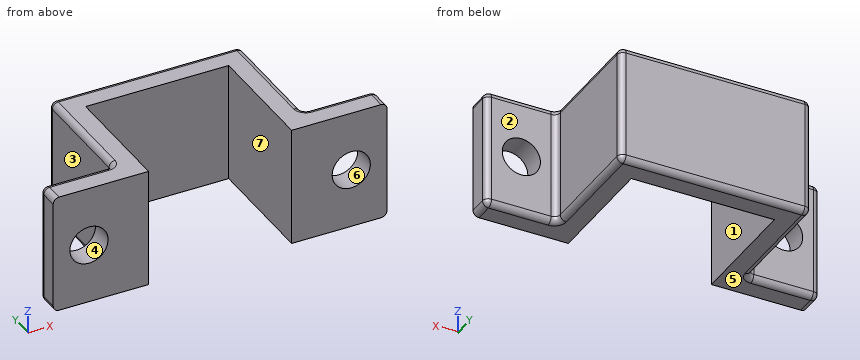
```python
from build123d import *

# Parameters (mm, degrees)
GRUNDK_RPER_DEPTH      = 10
SKIZZE2_W              = 12
SKIZZE2_H              = 10
AUSSCHNITT_MITTE_DEPTH = 21.976176963
SKIZZE3_R              = 1.6
BOHRUNGEN_DEPTH        = 20.899748742
VERRUNDUNG1_R          = 0.5


with BuildPart() as part:
    # Skizze1 → Grundkörper (new body)
    with BuildSketch(Plane.XY):
        Polygon((14, 0), (-14, 0), (-14, 2), (-8, 2), (-8, 12), (8, 12), (8, 2), (14, 2), align=None)
    extrude(amount=GRUNDK_RPER_DEPTH)

    # Skizze2 → Ausschnitt_Mitte (cut, through all)
    with BuildSketch(Plane.XY.offset(10)):
        with Locations((0, 5)):
            Rectangle(SKIZZE2_W, SKIZZE2_H)
    extrude(amount=-AUSSCHNITT_MITTE_DEPTH, mode=Mode.SUBTRACT)

    # Skizze3 → Bohrungen (cut, through all)
    with BuildSketch(Plane(origin=(0, 2, 0), x_dir=(1, 0, 0), z_dir=(0, 1, 0))):
        with Locations(Location((-11, -5, 0), (0, 0, 270))):
            Circle(SKIZZE3_R)
        with Locations(Location((11, -5, 0), (0, 0, 90))):
            Circle(SKIZZE3_R)
    extrude(amount=-BOHRUNGEN_DEPTH, mode=Mode.SUBTRACT)

    # Verrundung1
    verrundung1_edges = [part.edges().sort_by_distance(p)[0] for p in [
        (0, 12, 10),
        (8, 7, 0),
        (11, 2, 0),
        (-8, 7, 10),
        (14, 2, 5),
        (-14, 2, 5),
        (-8, 2, 5),
        (-8, 12, 5),
        (8, 12, 5),
        (8, 2, 5),
        (-11, 2, 10),
        (-14, 1, 10),
        (14, 1, 10),
        (11, 2, 10),
        (8, 7, 10),
        (14, 1, 0),
        (-14, 1, 0),
        (-11, 2, 0),
        (-8, 7, 0),
        (0, 12, 0),
    ]]
    fillet(verrundung1_edges, radius=VERRUNDUNG1_R)


solid = part.part
```
For this review, take the finished solid that the model builds, in its own axes (mm). Face numbers are marked on the shaded views. A direction names the side the tool comes from. Round coordinates to 2 decimals unless told otherwise and drop trailing zeros. Write each loop counter-clockwise with the first axis right and the second up, starting at its lowest first coordinate (ties: lowest second). Pieces come first, ordered by that corner, then holes. Notation, with made-up numbers: (6, 64) - (29, 64) arc R21 ccw to (29, 83) - close; hole circle Ø6 at (32, -23). An arc over 180 degrees is marked (long way). Write each question's results on one line, items separated by ' | '.
Item 1: Take a section at C-C on y = 3.5. State the section outline as (x, z) points, then the cut area to 3 significant figures.
Calculated:
outline: (-8, 0.5) arc R0.5 ccw to (-7.5, 0) - (-6, 0) - (-6, 10) - (-7.5, 10) arc R0.5 ccw to (-8, 9.5) - close; (6, 0) - (7.5, 0) arc R0.5 ccw to (8, 0.5) - (8, 9.5) arc R0.5 ccw to (7.5, 10) - (6, 10) - close | area: 39.8 mm^2
Item 2: To check wall thickness, follow line 1 along X through (y, z) = (1.5, 5); line 2 along Z through (x, y) = (11, 0.65); line 3 along X through (y, z) = (5, 3.75). State the ranges of each line that lie inside material, in increasing order. Write a range as from..to.
Calculated:
line 1: x = -14..-12.6, -9.4..-6, 6..9.4, 12.6..14 | line 2: z = 0..3.4, 6.6..10 | line 3: x = -8..-6, 6..8
Item 3: Take a section at A-A on x = 11. State the section outline as (y, z) points.
Calculated:
outline: (0, 0) - (1.5, 0) arc R0.5 ccw to (2, 0.5) - (2, 3.4) - (0, 3.4) - close; (0, 6.6) - (2, 6.6) - (2, 9.5) arc R0.5 ccw to (1.5, 10) - (0, 10) - close
Item 4: For the marked faces 1, 2, 3 and 4, list the 3-axis set-ups (+Z, -Z, +X, -X, +Y, -Y) from which the entire face can be reached by the end or side of a thin tool; tool diameter is ignored.
Calculated:
face 1: +Z, -Z, -Y | face 2: +Z, -Z, +X, +Y | face 3: +Z, -Z, -X, +Y | face 4: +Y, -Y
Item 5: Draft analysis for pull direction Z (two halves, no side actions). For the marked faces 5, 6 and 7, state which applies: pulls with the +Z half, pulls with the -Z half, needs draft (parallel to the pull), parting line crosses it, or undercut.
Calculated:
face 5: pulls with the -Z half | face 6: undercut | face 7: needs draft
Item 6: For pin 1 (1.5 mm diameter, centred on x = -10, z = 7, fed in from +Y); pin 2 (6 mm diameter, centred on x = 0.5, z = 5, fed in from -Y); pin 3 (3 mm diameter, centred on y = 3, z = 3.5, fed in from +X); pin 4 (2 mm diameter, centred on y = 9, z = 7, fed in from -X), all flat-tipped, find the tip position at first contact; note any pin that passes through.
Calculated:
pin 1: stops at y = 2 | pin 2: stops at y = 10 | pin 3: stops at x = 14 | pin 4: stops at x = -8
Item 7: Take a section at D-D on z = 2. State the section outline as (x, y) points, then the cut area to 3 significant figures.
Calculated:
outline: (-14, 0) - (-6, 0) - (-6, 10) - (6, 10) - (6, 0) - (14, 0) - (14, 1.5) arc R0.5 ccw to (13.5, 2) - (8.5, 2) arc R0.5 cw to (8, 2.5) - (8, 11.5) arc R0.5 ccw to (7.5, 12) - (-7.5, 12) arc R0.5 ccw to (-8, 11.5) - (-8, 2.5) arc R0.5 cw to (-8.5, 2) - (-13.5, 2) arc R0.5 ccw to (-14, 1.5) - close | area: 95.9 mm^2
Item 8: Take a section at B-B on z = 5. State the section outline as (x, y) points.
Calculated:
outline: (-14, 0) - (-12.6, 0) - (-12.6, 2) - (-13.5, 2) arc R0.5 ccw to (-14, 1.5) - close; (-9.4, 0) - (-6, 0) - (-6, 10) - (6, 10) - (6, 0) - (9.4, 0) - (9.4, 2) - (8.5, 2) arc R0.5 cw to (8, 2.5) - (8, 11.5) arc R0.5 ccw to (7.5, 12) - (-7.5, 12) arc R0.5 ccw to (-8, 11.5) - (-8, 2.5) arc R0.5 cw to (-8.5, 2) - (-9.4, 2) - close; (12.6, 0) - (14, 0) - (14, 1.5) arc R0.5 ccw to (13.5, 2) - (12.6, 2) - close
